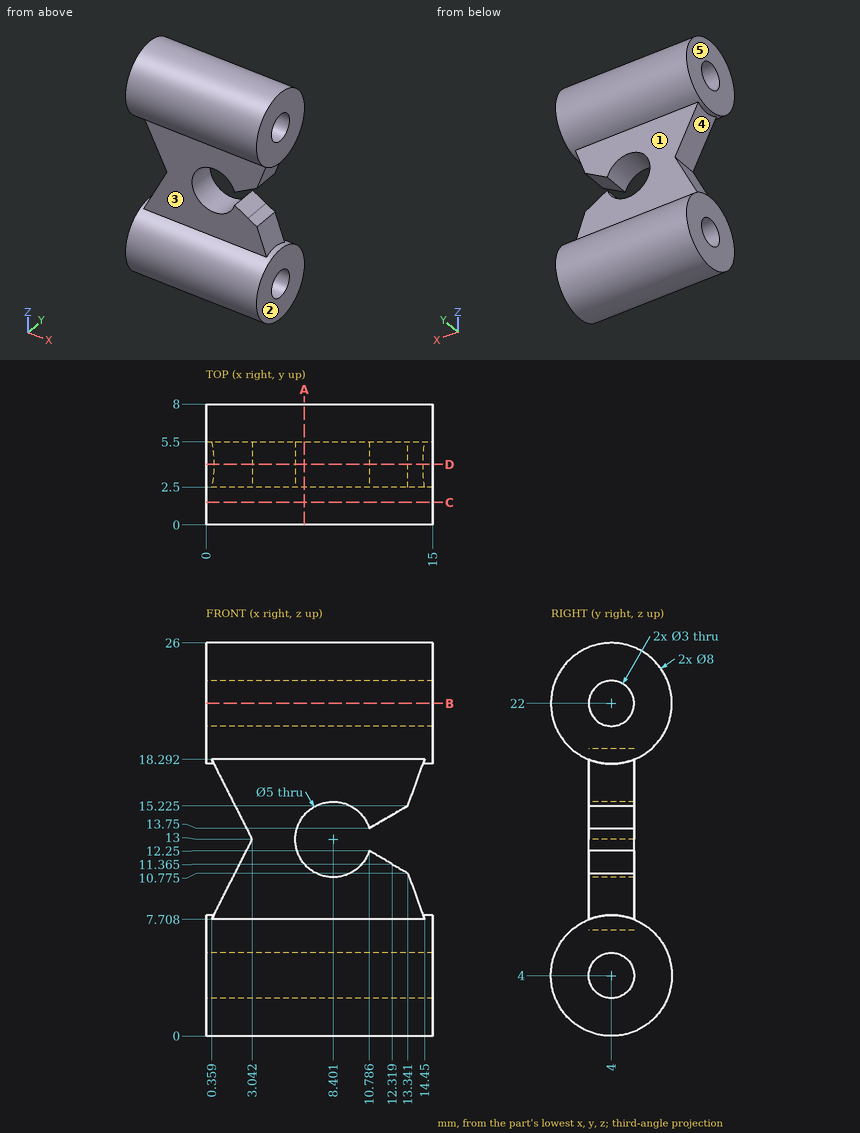
Job drawing, mm, ordinate dimensions from the low corner. One solid piece. A direction names the side the tool comes from. Round coordinates to 2 decimals unless told otherwise and drop trailing zeros. Loops run counter-clockwise (first coordinate to the right, second up) from the corner with the lowest first, then second, coordinate; pieces in that order, holes last.
(1) Two-plate mould, pull along Z, no slides. Class the marked faces 4 and 5: +Z half, -Z half, draft (parallel to the pull), parting line (faces both ways), or undercut.
(2) Which spindle directions (+Z, -Z, +X, -X, +Y, -Y) get a long thin tool onto all of the face, cutting with end or side? Do the marked faces 1, 2 and 3. Say none if no direction does.
(3) Cut at B-B (z = 22). Give the cut face in (x, y).
(4) Drop flat-ended pins along their axis: pin 1 (3 mm diameter, centred on x = 10, z = 14, fed in from -Y); pin 2 (5 mm diameter, centred on x = 11.5, z = 19, fed in from -Y); pin 3 (1.5 mm diameter, centred on x = 9.5, y = 5.5, fed in from -Z). Give the stop position or say it passes through.
(5) Cut at C-C (y = 1.5). Give the cut face in (x, z).
(6) Cut at D-D (y = 4). State how many separate pieces and enclosed holes the cut face has, plus the area to 3 significant figures.
(7) Wall check: line 1 along Z through (x, y) = (4.5, 4); line 2 along Y through (x, z) = (6.25, 4); line 3 along Z through (x, y) = (13.25, 4.25). Give the ranges that are in metal, low to high.
(8) Cut at A-A (x = 6.5). Give the cut face in (y, z), plus the area to 3 significant figures.
Findings below:
1. face 4: undercut
1. face 5: draft
2. face 1: +X, -X, +Y
2. face 2: +Z, -Z, +X, +Y, -Y
2. face 3: +X, -X, -Y
3. outline: (0, 0) - (15, 0) - (15, 2.5) - (0, 2.5) - close; (0, 5.5) - (15, 5.5) - (15, 8) - (0, 8) - close
4. pin 1: stops at y = 2.5
4. pin 2: stops at y = 0.03
4. pin 3: stops at z = 0.07
5. outline: (0, 0.88) - (15, 0.88) - (15, 7.12) - (0, 7.12) - close; (0, 18.88) - (15, 18.88) - (15, 25.12) - (0, 25.12) - close
6. separate pieces: 3
6. enclosed holes: 0
6. area: 241 mm2
7. line 1: z = 0 to 2.5, 5.5 to 20.5, 23.5 to 26
7. line 2: y = 0 to 2.5, 5.5 to 8
7. line 3: z = 0.01 to 2.52, 5.48 to 10.83, 15.17 to 20.52, 23.48 to 25.99
8. outline: (2.5, 7.71) arc R4 ccw (long way) to (5.5, 7.71) - (5.5, 11.38) - (2.5, 11.38) - close; (2.5, 14.62) - (5.5, 14.62) - (5.5, 18.29) arc R4 ccw (long way) to (2.5, 18.29) - close; hole circle Ø3 at (4, 4); hole circle Ø3 at (4, 22)
8. area: 107 mm2
